Autodesk Inventor part; units mm, degrees
ref_plane "YZ Plane" through (0, 0, 0) normal (1, 0, 0) x (0, 1, 0)
ref_plane "XZ Plane" through (0, 0, 0) normal (0, 1, 0) x (-1, 0, 0)
ref_plane "XY Plane" through (0, 0, 0) normal (0, 0, 1) x (1, 0, 0)
sketch "Sketch1" plane through (0, 0, 0) normal (0, 0, 1) x (1, 0, 0)
  line L0 (0, 0) -> (-107, 0)
  line L1 (-107, 0) -> (-107, 135)
  line L2 (-107, 135) -> (-115, 135)
  line L3 (-115, 135) -> (-115, 145)
  line L4 (-115, 145) -> (-119, 145)
  line L5 (-119, 145) -> (-119, 135)
  line L6 (-119, 135) -> (-127, 135)
  line L7 (-127, 135) -> (-127, 155)
  arc A0 (-119, 163) -> (-127, 155) centre (-119, 155) ccw
  line L8 (-119, 163) -> (0, 163)
  line L9 (0, 163) -> (0, 0)
  circle A1 centre (-119, 155) radius 2.5
  line L10 (-122.5, 142) -> (-121, 142)
  line L11 (-121, 142) -> (-121, 138)
  line L12 (-121, 138) -> (-122.5, 138)
  line L13 (-122.5, 138) -> (-122.5, 142)
  line L14 (-113, 142) -> (-111.5, 142)
  line L15 (-111.5, 142) -> (-111.5, 138)
  line L16 (-111.5, 138) -> (-113, 138)
  line L17 (-113, 138) -> (-113, 142)
  line L18 (-87, 147) -> (-52, 147)
  line L19 (-52, 147) -> (-52, 107)
  line L20 (-52, 107) -> (-87, 107)
  line L21 (-87, 107) -> (-87, 147)
  point P0 (-117, 145)
  point P1 (-121, 140)
  point P2 (-119, 140)
  point P3 (-113, 140)
  point P4 (-115, 140)
  point P5 (-52, 127)
  dimension "d1" = 145
  dimension "d3" = 4
  dimension "d4" = 10
  dimension "d5" = 10
  dimension "d6" = 10
  dimension "d7" = 127
  dimension "d8" = 8
  dimension "d9" = 10
  dimension "d10" = 5
  dimension "d14" = 4
  dimension "d15" = 8
  dimension "d16" = 1.5
  dimension "d17" = 4
  dimension "d18" = 40
  dimension "d19" = 35
  dimension "d20" = 127
  dimension "d21" = 20
extrude "Extrusion1" add sketch "Sketch1" along normal blind 6.477
fillet "Fillet1" radius 2 2 edges at (-107, 135, 3.2385) (-127, 135, 3.2385)
mirror "Mirror1" about plane through (-107, 0, 0) normal (0, -1, 0) of "Extrusion1", "Fillet1"
mirror "Mirror2" about plane through (0, 0, 0) normal (1, 0, 0) of "Extrusion1", "Mirror1", "Fillet1"
sketch "Sketch2" plane through (0, 0, 6.477) normal (0, 0, 1) x (1, 0, 0)
  arc A0 (5, 118) -> (10, 113) centre (10, 118) ccw
  line L0 (10, 113) -> (113, 113)
  line L1 (113, 113) -> (113, -113)
  line L2 (113, -113) -> (-113, -113)
  line L3 (-113, -113) -> (-113, 113)
  line L4 (-113, 113) -> (-10, 113)
  arc A1 (-10, 113) -> (-5, 118) centre (-10, 118) ccw
  line L5 (-5, 118) -> (-5, 142)
  arc A2 (5, 142) -> (-5, 142) centre (0, 142) ccw
  line L6 (5, 142) -> (5, 118)
  line L7 (-52, 147) -> (-52, 127)
  line L8 (-52, 127) -> (-87, 127)
  line L9 (-87, 127) -> (-87, 147)
  line L10 (-87, 147) -> (-52, 147)
  line L11 (-52, -147) -> (-87, -147)
  line L12 (-87, -147) -> (-87, -127)
  line L13 (-87, -127) -> (-52, -127)
  line L14 (-52, -127) -> (-52, -147)
  line L15 (52, 147) -> (87, 147)
  line L16 (87, 147) -> (87, 127)
  line L17 (87, 127) -> (52, 127)
  line L18 (52, 127) -> (52, 147)
  line L19 (52, -147) -> (52, -127)
  line L20 (52, -127) -> (87, -127)
  line L21 (87, -127) -> (87, -147)
  line L22 (87, -147) -> (52, -147)
  circle A3 centre (-119, 155) radius 2.5
  circle A4 centre (-119, -155) radius 2.5
  circle A5 centre (119, 155) radius 2.5
  circle A6 centre (119, -155) radius 2.5
  line L23 (-121, 138) -> (-122.5, 138)
  line L24 (-122.5, 138) -> (-122.5, 142)
  line L25 (-122.5, 142) -> (-121, 142)
  line L26 (-121, 142) -> (-121, 138)
  line L27 (-111.5, 138) -> (-113, 138)
  line L28 (-113, 138) -> (-113, 142)
  line L29 (-113, 142) -> (-111.5, 142)
  line L30 (-111.5, 142) -> (-111.5, 138)
  line L31 (-111.5, -142) -> (-113, -142)
  line L32 (-113, -142) -> (-113, -138)
  line L33 (-113, -138) -> (-111.5, -138)
  line L34 (-111.5, -138) -> (-111.5, -142)
  line L35 (-121, -142) -> (-122.5, -142)
  line L36 (-122.5, -142) -> (-122.5, -138)
  line L37 (-122.5, -138) -> (-121, -138)
  line L38 (-121, -138) -> (-121, -142)
  line L39 (111.5, 142) -> (113, 142)
  line L40 (113, 142) -> (113, 138)
  line L41 (113, 138) -> (111.5, 138)
  line L42 (111.5, 138) -> (111.5, 142)
  line L43 (121, 142) -> (122.5, 142)
  line L44 (122.5, 142) -> (122.5, 138)
  line L45 (122.5, 138) -> (121, 138)
  line L46 (121, 138) -> (121, 142)
  line L47 (111.5, -138) -> (113, -138)
  line L48 (113, -138) -> (113, -142)
  line L49 (113, -142) -> (111.5, -142)
  line L50 (111.5, -142) -> (111.5, -138)
  line L51 (121, -138) -> (122.5, -138)
  line L52 (122.5, -138) -> (122.5, -142)
  line L53 (122.5, -142) -> (121, -142)
  line L54 (121, -142) -> (121, -138)
  line L55 (-127, 155) -> (-127, -155)
  arc A7 (-127, -155) -> (-119, -163) centre (-119, -155) ccw
  line L56 (-119, -163) -> (119, -163)
  arc A8 (119, -163) -> (127, -155) centre (119, -155) ccw
  line L57 (127, -155) -> (127, 155)
  arc A9 (127, 155) -> (119, 163) centre (119, 155) ccw
  line L58 (119, 163) -> (-119, 163)
  arc A10 (-119, 163) -> (-127, 155) centre (-119, 155) ccw
  line L59 (-12.5, 113) -> (-12.5, 100.5)
  arc A11 (-12.5, 100.5) -> (12.5, 100.5) centre (0, 100.5) ccw
  line L60 (12.5, 100.5) -> (12.5, 113)
  point P0 (0, 0)
  dimension "d22" = 12.5
  dimension "d24" = 12.5
extrude "Extrusion2" cut sketch "Sketch2" against normal through all contours A0 L0 L60 A11 L59 L4 A1 L5 A2 L6
properties part number "BED PLATE BOTTOM"
Geometry: final body of the model. Coordinates: model frame, mm. A direction names the side the tool comes from. Coordinates: 2 decimals unless noted, no trailing zeros. Order: outer loops, then holes, each group sorted by start corner. A loop starts at its lowest first (then second) coordinate and runs counter-clockwise, first axis right, second up. Notation, with made-up numbers: M 35.25,-8.75 L 57.25,-8.75 A4 cw 57.25,-2.75 Z; hole C 59.5,-11.75 d11. An arc over 180 degrees is marked long. Answer in a Markdown table with one row per item. Add a question column.
Q1. Section query C-C on x = 0. Return the cut outline in (y, z), and give its area (3 significant figures).
Q2. Line query: L1, parallel to X at y = 155, z = 4.75; L2, parallel to Y at x = 112.5, z = 0.5; L3, parallel to X at y = -109.5, z = 3.25. Output: solid intervals per line, ascending.
Q3. Mould query, pull axis Y, two halves, no side actions, for faces 1 (the flat face through (2, -163, 3)), 2 (the flat face through (127, 146, 3)), 3 (the flat face through (87, 127, 3)). Classes: released by +Y, released by -Y, zero draft, split by the parting line, or undercut.
Q4. Reachability of faces 4 (the flat face through (69, 147, 3)), 5 (the flat face through (2, -2, 0)) from +Z, -Z, +X, -X, +Y, -Y: full face, straight path, thin tool, end or side. Return the list, or none.
Q5. Section query A-A on x = -66. Return the cut outline in (y, z), and give its area (3 significant figures).
Q6. Section query B-B on y = -117. Return the cut outline in (x, z), and give its area (3 significant figures).
Q7. Section query D-D on z = 2.5. Count the separate pieces of the cut face and the enclosed holes in it, and give its area (3 significant figures).
Q8. Contact query for flat-ended pins moving along their axis: P1, Ø1.6, axis at x = -121.5, z = 2.5, coming from the +Y side; P2, Ø1.8, axis at x = 121, z = 2, coming from the -Y side; P3, Ø2, axis at y = 92.5, z = 5, coming from the -X side. Output: stop coordinate, or through.
Completed:
| question | item | result |
|---|---|---|
| 1 | outline | M -163,0 L 88,0 L 88,6.48 L -163,6.48 Z; M 147,0 L 163,0 L 163,6.48 L 147,6.48 Z |
| 1 | area | 1,730 mm2 |
| 2 | L1 | x = -127 to -121.5, -116.5 to 116.5, 121.5 to 127 |
| 2 | L2 | y = -163 to -142, -138 to -135, 135 to 138, 142 to 163 |
| 2 | L3 | x = -107 to -87, -52 to 52, 87 to 107 |
| 3 | face 1 | released by -Y |
| 3 | face 2 | zero draft |
| 3 | face 3 | undercut |
| 4 | face 4 | +Z, -Z |
| 4 | face 5 | -Z, +X, -X, +Y, -Y |
| 5 | outline | M -163,0 L -147,0 L -147,6.48 L -163,6.48 Z; M -107,0 L 107,0 L 107,6.48 L -107,6.48 Z; M 147,0 L 163,0 L 163,6.48 L 147,6.48 Z |
| 5 | area | 1,590 mm2 |
| 6 | outline | M -107,0 L -87,0 L -87,6.48 L -107,6.48 Z; M -52,0 L 52,0 L 52,6.48 L -52,6.48 Z; M 87,0 L 107,0 L 107,6.48 L 87,6.48 Z |
| 6 | area | 933 mm2 |
| 7 | separate pieces | 1 |
| 7 | enclosed holes | 17 |
| 7 | area | 65,200 mm2 |
| 8 | P1 | stops at y = 162.82 |
| 8 | P2 | stops at y = -162.92 |
| 8 | P3 | stops at x = -107 |
